from build123d import *

# Parameters (mm, degrees)
CROQUIS1_W              = 70
CROQUIS1_H              = 70
CROQUIS1_R              = 2.5
SALIENTE_EXTRUIR1_DEPTH = 3
CORTAR_EXTRUIR1_REACH   = 5
CROQUIS2_R              = 2.1


with BuildPart() as part:
    # Croquis1 → Saliente-Extruir1 (new body)
    with BuildSketch(Plane.XY):
        Rectangle(CROQUIS1_W, CROQUIS1_H)
        with Locations((0, 25.4)):
            Circle(CROQUIS1_R, mode=Mode.SUBTRACT)
        with Locations((0, -25.4)):
            Circle(CROQUIS1_R, mode=Mode.SUBTRACT)
    extrude(amount=SALIENTE_EXTRUIR1_DEPTH)

    # Croquis2 → Cortar-Extruir1 (cut, up to next)
    with BuildSketch(Plane.XY.offset(3), mode=Mode.PRIVATE) as cortar_extruir1_sk1:
        with Locations((-12.7, 0)):
            Circle(CROQUIS2_R)
    cortar_extruir1_tool1 = extrude(cortar_extruir1_sk1.sketch, amount=-CORTAR_EXTRUIR1_REACH, mode=Mode.PRIVATE) & part.part
    add(cortar_extruir1_tool1.solids().sort_by_distance((-12.7, 0, 3))[0], mode=Mode.SUBTRACT)
    # Croquis2 → Cortar-Extruir1 (cut, up to next)
    with BuildSketch(Plane.XY.offset(3), mode=Mode.PRIVATE) as cortar_extruir1_sk2:
        with Locations((12.7, 0)):
            Circle(CROQUIS2_R)
    cortar_extruir1_tool2 = extrude(cortar_extruir1_sk2.sketch, amount=-CORTAR_EXTRUIR1_REACH, mode=Mode.PRIVATE) & part.part
    add(cortar_extruir1_tool2.solids().sort_by_distance((12.7, 0, 3))[0], mode=Mode.SUBTRACT)


solid = part.part
For this review, take the finished solid that the model builds, in its own axes (mm). Give positions to 0.01 mm unless a question says otherwise; leave off trailing zeros. Loops run counter-clockwise (first coordinate to the right, second up) from the corner with the lowest first, then second, coordinate; pieces in that order, holes last. Notation, with made-up numbers: (-38, -23) -> (-14, -23) arc R19 ccw to (-14, 3) -> close; hole circle Ø3 at (35, -2.5). An arc over 180 degrees is marked (long way). One line per question, with ' | ' between items.
1) To check wall thickness, follow probe 1 along Y at (x, z) = (0, 1.15); probe 2 along X at (y, z) = (1.5, 2.75); probe 3 along X at (y, z) = (-1, 1.3). State the ranges of each line that lie inside material, in increasing order.
Resolved:
probe 1: y = -35 to -27.9, -22.9 to 22.9, 27.9 to 35 | probe 2: x = -35 to -14.17, -11.23 to 11.23, 14.17 to 35 | probe 3: x = -35 to -14.55, -10.85 to 10.85, 14.55 to 35
2) We need section B-B (y = -25.4). Write out the cut boundary in (x, z).
Resolved:
outline: (-35, 0) -> (-2.5, 0) -> (-2.5, 3) -> (-35, 3) -> close; (2.5, 0) -> (35, 0) -> (35, 3) -> (2.5, 3) -> close
3) We need section A-A (x = 0). Write out the cut boundary in (y, z), plus the area to 3 significant figures.
Resolved:
outline: (-35, 0) -> (-27.9, 0) -> (-27.9, 3) -> (-35, 3) -> close; (-22.9, 0) -> (22.9, 0) -> (22.9, 3) -> (-22.9, 3) -> close; (27.9, 0) -> (35, 0) -> (35, 3) -> (27.9, 3) -> close | area: 180 mm2
4) The part is to be moulded in two halves that separate along Y. For faces 1 (the flat face through (-35, 0, 1)), 2 (the flat face through (0, -35, 1)), 3 (the cylindrical face through (-0.33, 27.88, 1.48)), say which applies: +Y half, -Y half, draft (parallel to the pull), parting line (faces both ways), or undercut.
Resolved:
face 1: draft | face 2: -Y half | face 3: undercut
5) We need section C-C (y = 0). Write out the cut boundary in (x, z).
Resolved:
outline: (-35, 0) -> (-14.8, 0) -> (-14.8, 3) -> (-35, 3) -> close; (-10.6, 0) -> (10.6, 0) -> (10.6, 3) -> (-10.6, 3) -> close; (14.8, 0) -> (35, 0) -> (35, 3) -> (14.8, 3) -> close
6) Insertion check: pin 1 Ø3 at (x, y) = (0, -25.4) entering from -Z. The pin has a flat end and moves straight along its axis. Give the tip position at first contact, or say it passes through.
Resolved:
pin 1: passes through
7) We need section D-D (x = -12.7). Write out the cut boundary in (y, z), plus the area to 3 significant figures.
Resolved:
outline: (-35, 0) -> (-2.1, 0) -> (-2.1, 3) -> (-35, 3) -> close; (2.1, 0) -> (35, 0) -> (35, 3) -> (2.1, 3) -> close | area: 197 mm2
